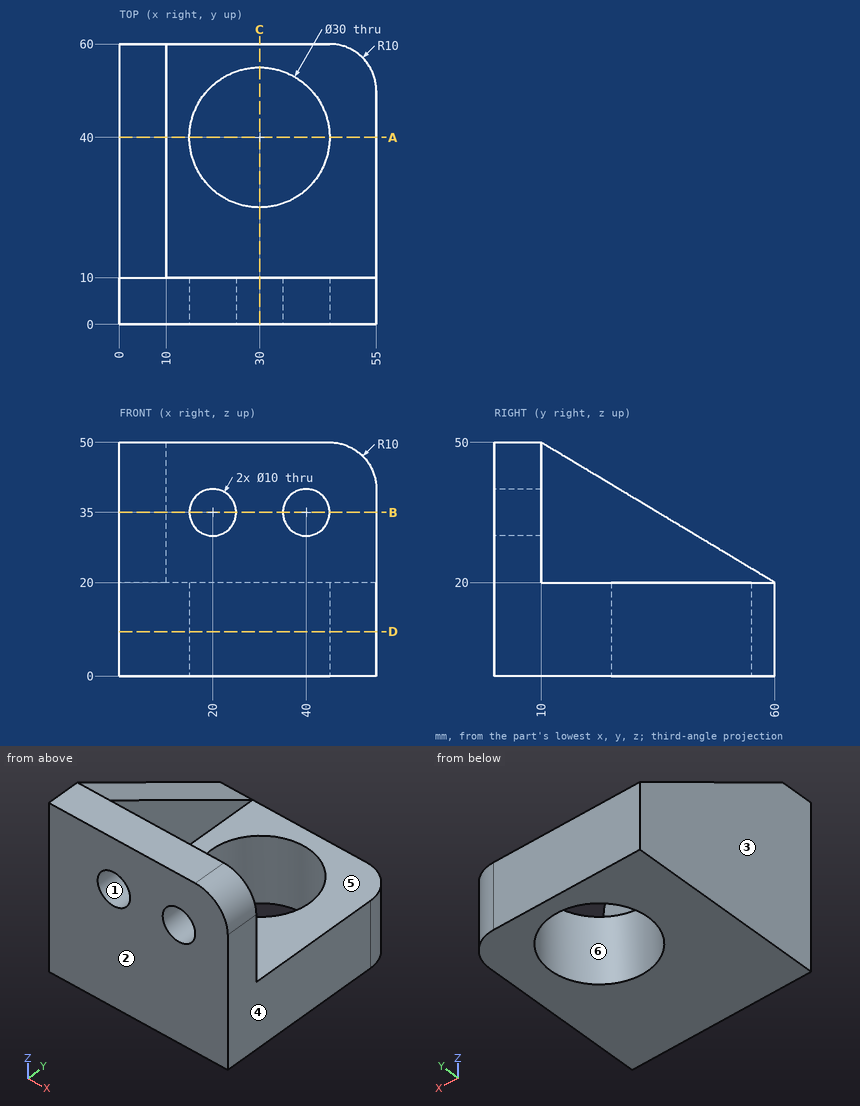
Here's the drawing with two shaded views (mm, measured from the low corner). I have some questions. A direction names the side the tool comes from. Give positions to 0.01 mm unless a question says otherwise; leave off trailing zeros. Loops run counter-clockwise (first coordinate to the right, second up) from the corner with the lowest first, then second, coordinate; pieces in that order, holes last. Notation, with made-up numbers: (38, -19.75) - (67, -19.75) arc R18 ccw to (67, 13.25) - close; hole circle Ø2 at (24, 80.25). An arc over 180 degrees is marked (long way). One line per item, written item: value.
(1) If we section it at C-C, the plane x = 30: List the corners of the cut face in (y, z) for me, plus the area to 3 significant figures.
Verdict:
outline: (0, 0) - (25, 0) - (25, 20) - (10, 20) - (10, 50) - (0, 50) - close; (55, 0) - (60, 0) - (60, 20) - (55, 20) - close
area: 900 mm^2
(2) If we section it at A-A, the plane y = 40: List the corners of the cut face in (x, z) for me.
Verdict:
outline: (0, 0) - (15, 0) - (15, 20) - (10, 20) - (10, 32) - (0, 32) - close; (45, 0) - (55, 0) - (55, 20) - (45, 20) - close
(3) On a 3-axis mill with a long thin cutter (end or side, diameter ignored), from which of +Z, -Z, +X, -X, +Y, -Y can I reach the whole of each face in a straight line? I mean the marked faces 5 and 6. Say none if no direction works.
Verdict:
face 5: +Z, +X, +Y
face 6: +Z, -Z
(4) If we mould it in two halves opening along X, with no side actions, what happens to the marked faces 1, 2, 3 and 4? For each: released by +X, released by -X, zero draft, split by the parting line, or undercut.
Verdict:
face 1: undercut
face 2: zero draft
face 3: released by -X
face 4: released by +X
(5) If we section it at B-B, the plane z = 35: List the corners of the cut face in (x, y) for me, plus the area to 3 significant figures.
Verdict:
outline: (0, 0) - (15, 0) - (15, 10) - (10, 10) - (10, 35) - (0, 35) - close; (25, 0) - (35, 0) - (35, 10) - (25, 10) - close; (45, 0) - (55, 0) - (55, 10) - (45, 10) - close
area: 600 mm^2
(6) If we section it at D-D, the plane z = 9.5: List the corners of the cut face in (x, y) for me, plus the area to 3 significant figures.
Verdict:
outline: (0, 0) - (55, 0) - (55, 50) arc R10 ccw to (45, 60) - (0, 60) - close; hole circle Ø30 at (30, 40)
area: 2,570 mm^2
(7) I'm going to push flat-ended pins straight in: pin 1 (8 mm diameter, centred on x = 13, z = 39, fed in from -Y); pin 2 (12 mm diameter, centred on x = 30, z = 45, fed in from +Y). Where does each tip first touch, or does it pass through?
Verdict:
pin 1: y = 0
pin 2: y = 10
(8) I need wall thicknesses on line 1 along Z through (x, y) = (20, 5); line 2 along X through (y, z) = (6.75, 35); line 3 along X through (y, z) = (40, 5). Which ranges of each line are inside material? Lowest first, please.
Verdict:
line 1: 0 to 30, 40 to 50
line 2: 0 to 15, 25 to 35, 45 to 55
line 3: 0 to 15, 45 to 55
